Autodesk Inventor part; units mm, degrees
ref_plane "YZ Plane" through (0, 0, 0) normal (1, 0, 0) x (0, 1, 0)
ref_plane "XZ Plane" through (0, 0, 0) normal (0, 1, 0) x (-1, 0, 0)
ref_plane "XY Plane" through (0, 0, 0) normal (0, 0, 1) x (1, 0, 0)
sketch "Sketch1" plane through (0, 0, 0) normal (0, 0, 1) x (1, 0, 0)
  line L0 (-17.78, 0) -> (17.78, 0)
  line L1 (0, -17.78) -> (0, 17.78)
  line L2 (-12.7, 12.7) -> (12.7, 12.7)
  line L3 (12.7, 12.7) -> (12.7, -12.7)
  line L4 (12.7, -12.7) -> (-12.7, -12.7)
  line L5 (-12.7, -12.7) -> (-12.7, 12.7)
  line L6 (9.525, 9.525) -> (-9.525, 9.525)
  line L7 (-9.525, 9.525) -> (-9.525, -9.525)
  line L8 (-9.525, -9.525) -> (9.525, -9.525)
  line L9 (9.525, -9.525) -> (9.525, 9.525)
  point P0 (0, 0)
  point P1 (-12.7, 0)
  point P2 (0, 12.7)
  dimension "d0" = 25.4
  dimension "d1" = 3.175
extrude "Extrusion1" add sketch "Sketch1" along normal mid plane 304.8 contours L5 L2 L1 L6 L7 L0 | L0 L7 L8 L1 L4 L5 | L1 L8 L9 L0 L3 L4 | L2 L3 L0 L9 L6 L1
sketch "Sketch3" plane through (-12.7, 12.7, 152.4) normal (0, 1, 0) x (1, 0, 0)
  line L0 (0, 0) -> (25.4, 0)
  line L1 (25.4, 0) -> (25.4, 304.8)
  line L2 (0, 0) -> (25.4, 14.6647)
  point P0 (12.7, 152.4)
  dimension "d7" = 30
extrude "Extrusion3" cut sketch "Sketch3" against normal through all
sketch "Sketch4" plane through (-12.7, 12.7, -152.4) normal (0, 1, 0) x (1, 0, 0)
  line L0 (25.4, 0) -> (0, 0)
  line L1 (0, 0) -> (0, -304.8)
  line L2 (25.4, 0) -> (0, -14.6647)
  point P0 (12.7, -152.4)
  dimension "d10" = 30
extrude "Extrusion4" cut sketch "Sketch4" against normal through all
properties part number "tubing_template_0.125" material "Aluminum-6061"
For this review, take the finished solid that the model builds, in its own axes (mm). A direction names the side the tool comes from. Round coordinates to 2 decimals unless told otherwise and drop trailing zeros. Order: outer loops, then holes, each group sorted by start corner. A loop starts at its lowest first (then second) coordinate and runs counter-clockwise, first axis right, second up. Notation, with made-up numbers: (68.25, -9) -> (93.25, -9) arc R17 ccw to (93.25, 6) -> close; hole circle Ø5 at (4.5, 22.5). An arc over 180 degrees is marked (long way). Put each result on its own line as item: value.
Q1. Insertion check: pin 1 Ø12 at (x, y) = (8.5, 4) entering from +Z; pin 2 Ø3 at (x, y) = (-7.5, 8.5) entering from -Z. Each pin has a flat end and moves straight along its axis. Give the tip position at first contact, or say it passes through.
Check result:
pin 1: z = 141.51
pin 2: z = -141.37
Q2. Mouldability with a two-part tool opening along X and no side actions: class faces 1 (the flat face through (0, -12.7, -2)), 2 (the flat face through (-9.525, 0, 3)), 3 (the flat face through (0.18, -11.11, -145.17)) as pulls with the +X half, pulls with the -X half, needs draft (parallel to the pull), parting line crosses it, or undercut.
Check result:
face 1: needs draft
face 2: undercut
face 3: pulls with the -X half
Q3. Add section C-C on x = 1.5. Write out the cut boundary in (y, z) (3 decimals), plus the area to 3 significant figures.
Check result:
outline: (-12.7, -145.934) -> (-9.525, -145.934) -> (-9.525, 144.202) -> (-12.7, 144.202) -> close; (9.525, -145.934) -> (12.7, -145.934) -> (12.7, 144.202) -> (9.525, 144.202) -> close
area: 1,840 mm2
Q4. Add section A-A on y = 3. Write out the cut boundary in (x, z) (3 decimals).
Check result:
outline: (-12.7, -137.735) -> (-9.525, -139.568) -> (-9.525, 150.567) -> (-12.7, 152.4) -> close; (9.525, -150.567) -> (12.7, -152.4) -> (12.7, 137.735) -> (9.525, 139.568) -> close
Q5. Machinability: for faces 4 (the flat face through (-12.7, 0, 5)), 5 (the flat face through (9.525, 0, -8)), which of the approach directions +Z, -Z, +X, -X, +Y, -Y give a long, thin tool a straight path to every point of the face, cutting with its end or side? Answer none if there is none.
Check result:
face 4: +Z, -Z, -X, +Y, -Y
face 5: +Z, -Z
Q6. Add section B-B on z = -70. Write out the cut boundary in (x, y) (3 decimals), plus the area to 3 significant figures.
Check result:
outline: (-12.7, -12.7) -> (12.7, -12.7) -> (12.7, 12.7) -> (-12.7, 12.7) -> close; hole (-9.525, -9.525) -> (9.525, -9.525) -> (9.525, 9.525) -> (-9.525, 9.525) -> close
area: 282 mm2
Q7. For probe 1 along X at (y, z) = (-6.5, -72.5) (3 decimals); probe 2 along Z at (x, y) = (-10, 10.25), list the stretches that pass through material, from the lowest coordinate up. Write a range as [from, to].
Check result:
probe 1: [-12.7, -9.525], [9.525, 12.7]
probe 2: [-139.29, 150.84]
